```python
from build123d import *
from build123d.topology import SkipClean

# Parameters (mm, degrees)
EXTRUDE_1_DEPTH     = 200
SKETCH_2_W          = 10
SKETCH_2_H          = 180
CUT_EXTRUDE_1_DEPTH = 219.205820271
SKETCH_3_W          = 8
SKETCH_3_H          = 190
EXTRUDE_2_DEPTH     = 10
SKETCH_4_R          = 2.5
CUT_EXTRUDE_2_DEPTH = 214.632347738
SKETCH_5_W          = 20
SKETCH_5_H          = 3
EXTRUDE_3_DEPTH     = 10
CUT_EXTRUDE_3_DEPTH = 217.732046546
EXTRUDE_4_DEPTH     = 5
EXTRUDE_START       = 5
EXTRUDE_5_DEPTH     = 5
CUT_EXTRUDE_START   = -3
CUT_EXTRUDE_4_DEPTH = 3
CUT_EXTRUDE_5_DEPTH = 3


with BuildPart() as part:
    # 草圖1 → 填料-伸長1 (new body)
    with BuildSketch(Plane.XY):
        with BuildLine():
            Line((-61.7, 0), (-61.7, -10))
            Line((-61.7, -10), (-57.7, -10))
            Line((-57.7, -10), (-57.7, 0))
            ThreePointArc((-57.7, 0), (-2, 55.7), (53.7, 0))
            Line((53.7, 0), (61.7, 0))
            ThreePointArc((61.7, 0), (0, 61.7), (-61.7, 0))
        make_face()
    extrude(amount=EXTRUDE_1_DEPTH)

    # 草圖2 → 除料-伸長1 (cut, through all)
    with BuildSketch(Plane(origin=(0, 0, 0), x_dir=(1, 0, 0), z_dir=(0, 1, 0))):
        with Locations((0, -100)):
            Rectangle(SKETCH_2_W, SKETCH_2_H)
        with Locations((22, -100)):
            Rectangle(SKETCH_2_W, SKETCH_2_H)
        with Locations((44, -100)):
            Rectangle(SKETCH_2_W, SKETCH_2_H)
        with Locations((-21.943943619, -101.569502613)):
            Rectangle(SKETCH_2_W, SKETCH_2_H)
        with Locations((-43.887887238, -103.139005227)):
            Rectangle(SKETCH_2_W, SKETCH_2_H)
    extrude(amount=CUT_EXTRUDE_1_DEPTH, mode=Mode.SUBTRACT)

    # 草圖3 → 填料-伸長2 (add)
    with BuildSketch(Plane.XZ):
        with Locations((57.7, 100)):
            Rectangle(SKETCH_3_W, SKETCH_3_H)
    extrude(amount=EXTRUDE_2_DEPTH)

    # 草圖4 → 除料-伸長2 (cut, through all)
    with BuildSketch(Plane.XY.offset(195)):
        with Locations((57.7, -5)):
            Circle(SKETCH_4_R)
    extrude(amount=-CUT_EXTRUDE_2_DEPTH, mode=Mode.SUBTRACT)

    # 草圖5 → 填料-伸長3 (add)
    with BuildSketch(Plane.ZY.offset(61.7)):
        with Locations((100, -8.5)):
            Rectangle(SKETCH_5_W, SKETCH_5_H)
    extrude(amount=EXTRUDE_3_DEPTH)

    # 草圖6 → 除料-伸長3 (cut, through all)
    with BuildSketch(Plane.XY.offset(195)):
        Polygon((61.7, -10), (61.7, -6), (55.7, -10), align=None)
    extrude(amount=-CUT_EXTRUDE_3_DEPTH, mode=Mode.SUBTRACT)

    # 草圖7 → 填料-伸長4 (add)
    with SkipClean():  # the faces are left unmerged after this step: merging them gives an invalid solid
        with BuildSketch(Plane.XY.offset(200)):
            with BuildLine():
                Line((61.7, 0), (-61.7, 0))
                ThreePointArc((-61.7, 0), (0, 61.7), (61.7, 0))
            make_face()
        extrude(amount=EXTRUDE_4_DEPTH)

    # 草圖8 → 填料-伸長5 (add)
    with SkipClean():  # the faces are left unmerged after this step: merging them gives an invalid solid
        with BuildSketch(Plane(origin=(0, 0, 0), x_dir=(-1, 0, 0), z_dir=(0, 0, -1)).offset(EXTRUDE_START)):
            with BuildLine():
                Line((-61.7, 0), (61.7, 0))
                ThreePointArc((61.7, 0), (0, 61.7), (-61.7, 0))
            make_face()
        extrude(amount=-EXTRUDE_5_DEPTH)

    # 草圖9 → 除料-伸長4 (cut)
    with SkipClean():  # the faces are left unmerged after this step: merging them gives an invalid solid
        with BuildSketch(Plane.XY.offset(CUT_EXTRUDE_START)):
            with BuildLine():
                Line((-57.7, 0), (53.7, 0))
                ThreePointArc((53.7, 0), (-2, 55.7), (-57.7, 0))
            make_face()
        extrude(amount=CUT_EXTRUDE_4_DEPTH, mode=Mode.SUBTRACT)

    # 草圖10 → 除料-伸長5 (cut)
    with SkipClean():  # the faces are left unmerged after this step: merging them gives an invalid solid
        with BuildSketch(Plane(origin=(0, 0, 200), x_dir=(-1, 0, 0), z_dir=(0, 0, -1))):
            with BuildLine():
                Line((-53.7, 0), (57.7, 0))
                ThreePointArc((57.7, 0), (2, 55.7), (-53.7, 0))
            make_face()
        extrude(amount=-CUT_EXTRUDE_5_DEPTH, mode=Mode.SUBTRACT)


solid = part.part
```
Geometry: final body of the model. Coordinates: model frame, mm. A direction names the side the tool comes from. Coordinates: 2 decimals unless noted, no trailing zeros. Order: outer loops, then holes, each group sorted by start corner. A loop starts at its lowest first (then second) coordinate and runs counter-clockwise, first axis right, second up. Notation, with made-up numbers: (41, 23) - (46, 23) arc R19 cw to (46, 40) - close; hole circle Ø11 at (69.25, 56.25). An arc over 180 degrees is marked (long way). Write each question's results on one line, items separated by ' | '.
(1) Mould query, pull axis Y, two halves, no side actions, for faces 5 (the face through (55.2, -4.9, 101.3)), 6 (the face through (8.9, 0, 203.3)), 7 (the face through (-44, 39, 193.139)). Classes: +Y half, -Y half, draft (parallel to the pull), parting line (faces both ways), or undercut.
Values found:
face 5: undercut | face 6: -Y half | face 7: draft
(2) Set-up query: faces 1 (the face through (53.7, -5, 99)), 2 (the face through (-60, -5, 0)), 3 (the face through (-48.888, 34, 104)), 4 (the face through (-38.888, 45, 104)). Return all of +Z, -Z, +X, -X, +Y, -Y with unobstructed straight access to the full face (end or side cutting, diameter ignored); none if empty.
Values found:
face 1: +Z, -Z, -Y | face 2: -Z, +X, -X, -Y | face 3: +Y, -Y | face 4: -X, +Y, -Y
(3) Line query: line 1 (Z direction, x = -17.5, y = 25); line 2 (Z direction, x = -42, y = 41); line 3 (X direction, y = 26, z = 109). Output: solid intervals per line, ascending. Write a range as [from, to].
Values found:
line 1: z = [-5, -3], [203, 205] | line 2: z = [-5, 13.14], [193.14, 205] | line 3: x = [-55.95, -51.26], [49, 55.95]
(4) Section query B-B, the plane x = -2. Return the cut outline in (y, z).
Values found:
outline: (0, -5) - (61.67, -5) - (61.67, 10) - (55.7, 10) - (55.7, -3) - (0, -3) - close; (0, 203) - (55.7, 203) - (55.7, 190) - (61.67, 190) - (61.67, 205) - (0, 205) - close
(5) First-contact query: pin 1 Ø12 at (x, z) = (-57.5, 73.5) entering from +Y; pin 2 Ø6.5 at (y, z) = (60, 89.5) entering from +X; pin 3 Ø8 at (x, z) = (1.5, 201) entering from -Y. Flat tips, straight axial feed; report the tip coordinate or a pass-through.
Values found:
pin 1: stops at y = 33.98 | pin 2: stops at x = 17 | pin 3: stops at y = 0
(6) Section query A-A, the plane z = 184.5. Count the separate pieces of the cut face and the enclosed holes in it, plus the area to 3 significant figures.
Values found:
separate pieces: 6 | enclosed holes: 1 | area: 816 mm²
(7) Section query C-C, the plane x = 35. Return the cut outline in (y, z), plus the area to 3 significant figures.
Values found:
outline: (0, -5) - (50.81, -5) - (50.81, 205) - (0, 205) - (0, 203) - (41.64, 203) - (41.64, -3) - (0, -3) - close | area: 2,090 mm²
